```python
from build123d import *

# Parameters (mm, degrees)
ESQUISSE1_W             = 7
ESQUISSE1_H             = 4.3
BOSS_EXTRU_1_DEPTH      = 7.5
COQUE1_T                = -1
ESQUISSE2_W             = 1.25
ESQUISSE2_H             = 0.8
BOSS_EXTRU_2_DEPTH      = 3.1
ESQUISSE3_W             = 1.5
ESQUISSE3_H             = 0.8
BOSS_EXTRU_3_DEPTH      = 3.1
ESQUISSE4_R             = 0.14
ENL_V_MAT_EXTRU_1_DEPTH = 13.192210628
BOSS_EXTRU_4_DEPTH      = 1.25
BOSS_EXTRU_5_START      = -1.25
BOSS_EXTRU_5_DEPTH      = 1.25
BOSS_EXTRU_6_DEPTH      = 1.5
CONG_1_R                = 1


with BuildPart() as part:
    # Esquisse1 → Boss.-Extru.1 (new body)
    with BuildSketch(Plane(origin=(0, 0, 0), x_dir=(1, 0, 0), z_dir=(0, 1, 0))):
        with Locations((3.5, 2.15)):
            Rectangle(ESQUISSE1_W, ESQUISSE1_H)
    extrude(amount=BOSS_EXTRU_1_DEPTH)

    # Coque1
    coque1_openings = [part.faces().sort_by_distance(p)[0] for p in [
        (3.5, 0, -2.15),
    ]]
    offset(amount=COQUE1_T, openings=coque1_openings, kind=Kind.INTERSECTION)

    # Esquisse2 → Boss.-Extru.2 (add)
    with BuildSketch(Plane.XY):
        with Locations((1.125, 0.4)):
            Rectangle(ESQUISSE2_W, ESQUISSE2_H)
        with Locations((4.375, 0.4)):
            Rectangle(ESQUISSE2_W, ESQUISSE2_H)
    extrude(amount=BOSS_EXTRU_2_DEPTH)

    # Esquisse3 → Boss.-Extru.3 (add)
    with BuildSketch(Plane(origin=(0, 0, -4.3), x_dir=(-1, 0, 0), z_dir=(0, 0, -1))):
        with Locations((-4.75, 0.4)):
            Rectangle(ESQUISSE3_W, ESQUISSE3_H)
    extrude(amount=BOSS_EXTRU_3_DEPTH)

    # Esquisse4 → Enlèv. mat.-Extru.1 (cut, through all)
    with BuildSketch(Plane(origin=(0, 0.8, 0), x_dir=(1, 0, 0), z_dir=(0, 1, 0))):
        with Locations(Location((4.75, 6.75, 0), (0, 0, 270))):
            Circle(ESQUISSE4_R)
        with Locations(Location((1.125, -2.45, 0), (0, 0, 270))):
            Circle(ESQUISSE4_R)
        with Locations(Location((4.375, -2.45, 0), (0, 0, 270))):
            Circle(ESQUISSE4_R)
    extrude(amount=-ENL_V_MAT_EXTRU_1_DEPTH, mode=Mode.SUBTRACT)

    # Esquisse5 → Boss.-Extru.4 (add)
    with BuildSketch(Plane(origin=(5, 0, 0), x_dir=(0, 0, -1), z_dir=(1, 0, 0))):
        with BuildLine():
            Line((0, 2.5), (0, 0.8))
            Line((0, 0.8), (-1.7, 0.8))
            ThreePointArc((-1.7, 0.8), (-1.202081528, 2.002081528), (0, 2.5))
        make_face()
    extrude(amount=-BOSS_EXTRU_4_DEPTH)

    # Esquisse6 → Boss.-Extru.5 (add)
    with BuildSketch(Plane.ZY.offset(-0.5).offset(BOSS_EXTRU_5_START)):
        with BuildLine():
            Line((0, 2.5), (0, 0.8))
            Line((0, 0.8), (1.7, 0.8))
            ThreePointArc((1.7, 0.8), (1.202081528, 2.002081528), (0, 2.5))
        make_face()
    extrude(amount=BOSS_EXTRU_5_DEPTH)

    # Esquisse7 → Boss.-Extru.6 (add)
    with BuildSketch(Plane.ZY.offset(-4)):
        with BuildLine():
            Line((-4.3, 2.5), (-4.3, 0.8))
            Line((-4.3, 0.8), (-6, 0.8))
            ThreePointArc((-6, 0.8), (-5.502081528, 2.002081528), (-4.3, 2.5))
        make_face()
    extrude(amount=-BOSS_EXTRU_6_DEPTH)

    # Congé1
    # the kernel refuses this fillet: 1 mm, written as the material it takes off along each edge
    with BuildSketch(Plane(origin=(0, -2.5, 0), x_dir=(1, 0, 0), z_dir=(0, 1, 0))) as cong_1_piece_1_section:
        with BuildLine():
            CenterArc((CONG_1_R, CONG_1_R), CONG_1_R, 180, 90)
            Line((0, CONG_1_R), (0, 0))
            Line((0, 0), (CONG_1_R, 0))
        make_face()
    cong_1_piece_1 = extrude(amount=12.5, mode=Mode.PRIVATE)
    cong_1_piece_1 = split(cong_1_piece_1, bisect_by=Plane(origin=(0.5, 1.236097217, -0.241175313), z_dir=(-1, 0, 0)), keep=Keep.TOP, mode=Mode.PRIVATE)
    add(cong_1_piece_1, mode=Mode.SUBTRACT)
    with BuildSketch(Plane(origin=(0, -2.5, 0), x_dir=(1, 0, 0), z_dir=(0, 1, 0))) as cong_1_piece_2_section:
        with BuildLine():
            CenterArc((CONG_1_R, CONG_1_R), CONG_1_R, 180, 90)
            Line((0, CONG_1_R), (0, 0))
            Line((0, 0), (CONG_1_R, 0))
        make_face()
    cong_1_piece_2 = extrude(amount=12.5, mode=Mode.PRIVATE)
    cong_1_piece_2 = cong_1_piece_2 - Plane(origin=(0.623254318, 0.8, 0), x_dir=(0, 0, 1), z_dir=(1, 0, 0)) * Cylinder(1.7, 29, mode=Mode.PRIVATE)
    add(cong_1_piece_2, mode=Mode.SUBTRACT)
    with BuildSketch(Plane(origin=(0, -2.5, -4.3), x_dir=(1, 0, 0), z_dir=(0, 1, 0)), Plane(origin=(7, -2.5, -4.3), x_dir=(0, 0, 1), z_dir=(0, 1, 0)), Plane(origin=(7, -2.5, 0), x_dir=(-1, 0, 0), z_dir=(0, 1, 0))) as cong_1_piece_3:
        with BuildLine():
            CenterArc((CONG_1_R, -CONG_1_R), CONG_1_R, 90, 90)
            Line((0, -CONG_1_R), (0, 0))
            Line((0, 0), (CONG_1_R, 0))
        make_face()
    extrude(amount=12.5, mode=Mode.SUBTRACT)


solid = part.part
```
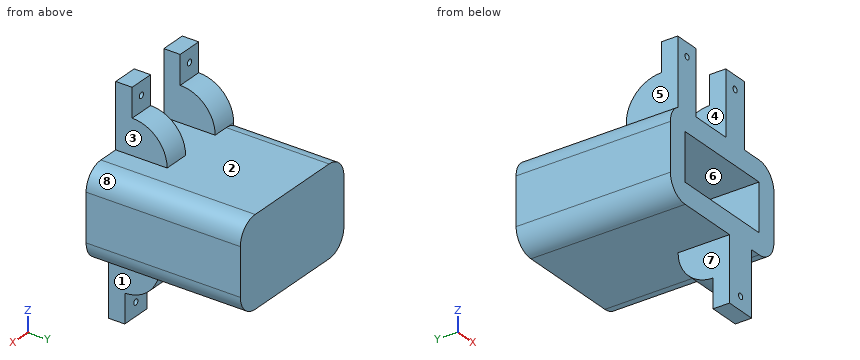
Can you work these out from the model? Positions are in its coordinate system, mm. Face numbers are marked on the shaded views. A direction names the side the tool comes from. Coordinates: 2 decimals unless noted, no trailing zeros. Loops run counter-clockwise (first coordinate to the right, second up) from the corner with the lowest first, then second, coordinate; pieces in that order, holes last.
Item 1: I'm going to push flat-ended pins straight in: pin 1 (2.5 mm diameter, centred on x = 2.5, y = 3.5, fed in from -Z); pin 2 (1.5 mm diameter, centred on x = 3.5, y = 3.5, fed in from +Z); pin 3 (0.8 mm diameter, centred on y = 1.5, z = 1.5, fed in from -X). Where does each tip first touch, or does it pass through?
Answers below:
pin 1: stops at z = -4.3
pin 2: stops at z = 0
pin 3: stops at x = 0.5
Item 2: Please list where these lines run through material, in increasing order: L1, parallel to X at y = 0.5, z = 2.45 (3 decimals); L2, parallel to Z at x = 4.5, y = 4.75; L3, parallel to X at y = 5.5, z = -2.75.
Answers below:
L1: x = 0.5 to 0.985, 1.265 to 1.75, 3.75 to 4.235, 4.515 to 5
L2: z = -4.3 to -3.3, -1 to 0
L3: x = 0 to 1, 6 to 7
Item 3: If we mould it in two halves opening along Z, with no side actions, what happens to the marked faces 6, 7 and 8? For each: released by +Z, released by -Z, zero draft, split by the parting line, or undercut.
Answers below:
face 6: undercut
face 7: zero draft
face 8: released by +Z
Item 4: Suppose I cut it at D-D (z = 2.45). Please give me the cut outline in (x, y) (3 decimals), then the cut area to 3 significant figures.
Answers below:
outline: (0.5, 0) - (0.985, 0) - (0.985, 0.8) - (0.5, 0.8) - close; (1.265, 0) - (1.75, 0) - (1.75, 0.8) - (1.265, 0.8) - close; (3.75, 0) - (4.235, 0) - (4.235, 0.8) - (3.75, 0.8) - close; (4.515, 0) - (5, 0) - (5, 0.8) - (4.515, 0.8) - close
area: 1.55 mm2
Item 5: Which directions (+Z, -Z, +X, -X, +Y, -Y) give clear straight access to the entire face, cutting with the end or side of a thin tool? Please do the marked faces 1, 2, 3, 4 and 5.
Answers below:
face 1: -Z, +X, +Y, -Y
face 2: +Z, +Y
face 3: +Z, +X, +Y, -Y
face 4: +Z, +Y, -Y
face 5: +Z, -X, +Y, -Y
Item 6: Suppose I cut it at B-B (x = 4.75). Please give me the cut outline in (y, z), then the cut area to 3 significant figures.
Answers below:
outline: (0, -7.4) - (0.8, -7.4) - (0.8, -6.89) - (0, -6.89) - close; (0, -6.61) - (0.8, -6.61) - (0.8, -6) arc R1.7 ccw to (2.5, -4.3) - (7.5, -4.3) - (7.5, 0) - (2.5, 0) arc R1.7 ccw to (0.8, 1.7) - (0.8, 3.1) - (0, 3.1) - (0, -1) - (6.5, -1) - (6.5, -3.3) - (0, -3.3) - close
area: 26.6 mm2
Item 7: Suppose I cut it at A-A (z = -6.75). Please give me the cut outline in (x, y), then the cut area to 3 significant figures.
Answers below:
outline: (4, 0) - (4.61, 0) - (4.61, 0.8) - (4, 0.8) - close; (4.89, 0) - (5.5, 0) - (5.5, 0.8) - (4.89, 0.8) - close
area: 0.976 mm2
Item 8: Suppose I cut it at C-C (y = 3.5). Please give me the cut outline in (x, z).
Answers below:
outline: (0, -3.3) arc R1 ccw to (1, -4.3) - (6, -4.3) arc R1 ccw to (7, -3.3) - (7, -1) arc R1 ccw to (6, 0) - (1, 0) arc R1 ccw to (0, -1) - close; hole (1, -3.3) - (6, -3.3) - (6, -1) - (1, -1) - close
